```python
from build123d import *

# Parameters (mm, degrees)
F0_R     = 3
F1_DEPTH = 2
F2_DEPTH = 4
F4_DEPTH = 2
F5_DEPTH = 3


with BuildPart() as f1:
    # F0 (on Top) → F1 (new body)
    with BuildSketch(Plane.XY):
        with Locations((-50.25617, 22.832299)):
            Circle(F0_R)
        with BuildLine():
            Line((-57, -28.5), (43, -28.5))
            ThreePointArc((43, -28.5), (44.414214, -27.914214), (45, -26.5))
            Line((45, -26.5), (45, 26.5))
            ThreePointArc((45, 26.5), (44.414214, 27.914214), (43, 28.5))
            Line((43, 28.5), (-57, 28.5))
            Line((-57, 28.5), (-57, -28.5))
        make_face()
        with Locations((-50.25617, 22.832299)):
            Circle(F0_R, mode=Mode.SUBTRACT)
        with BuildLine():
            ThreePointArc((44, -26.5), (43.707107, -27.207107), (43, -27.5))
            Line((43, -27.5), (-43, -27.5))
            ThreePointArc((-43, -27.5), (-43.707107, -27.207107), (-44, -26.5))
            Line((-44, -26.5), (-44, 26.5))
            ThreePointArc((-44, 26.5), (-43.707107, 27.207107), (-43, 27.5))
            Line((-43, 27.5), (43, 27.5))
            ThreePointArc((43, 27.5), (43.707107, 27.207107), (44, 26.5))
            Line((44, 26.5), (44, -26.5))
        make_face(mode=Mode.SUBTRACT)
        with BuildLine():
            Line((-43, -27.5), (43, -27.5))
            ThreePointArc((43, -27.5), (43.707107, -27.207107), (44, -26.5))
            Line((44, -26.5), (44, 26.5))
            ThreePointArc((44, 26.5), (43.707107, 27.207107), (43, 27.5))
            Line((43, 27.5), (-43, 27.5))
            ThreePointArc((-43, 27.5), (-43.707107, 27.207107), (-44, 26.5))
            Line((-44, 26.5), (-44, -26.5))
            ThreePointArc((-44, -26.5), (-43.707107, -27.207107), (-43, -27.5))
        make_face()
    extrude(amount=F1_DEPTH)

    # F0 (on Top) → F2 (join)
    with BuildSketch(Plane.XY):
        with BuildLine():
            ThreePointArc((45, -26.5), (44.414214, -27.914214), (43, -28.5))
            Line((43, -28.5), (-57, -28.5))
            Line((-57, -28.5), (-57, -31.5))
            Line((-57, -31.5), (43, -31.5))
            ThreePointArc((43, -31.5), (46.535534, -30.035534), (48, -26.5))
            Line((48, -26.5), (48, 26.5))
            ThreePointArc((48, 26.5), (46.535534, 30.035534), (43, 31.5))
            Line((43, 31.5), (-57, 31.5))
            Line((-57, 31.5), (-57, 28.5))
            Line((-57, 28.5), (43, 28.5))
            ThreePointArc((43, 28.5), (44.414214, 27.914214), (45, 26.5))
            Line((45, 26.5), (45, -26.5))
        make_face()
    extrude(amount=F2_DEPTH)

    # F3 (on face) → F4 (cut)
    with BuildSketch(Plane.XY.offset(4)):
        Polygon((45, 3), (45, 0), (45, -3), (48, -3), (48, 0), (48, 3), align=None)
    extrude(amount=-F4_DEPTH, mode=Mode.SUBTRACT)

    # F0 (on Top) → F5 (cut)
    with BuildSketch(Plane.XY):
        with Locations((-50.25617, 22.832299)):
            Circle(F0_R)
    extrude(amount=F5_DEPTH, mode=Mode.SUBTRACT)


solid = f1.part
```
Input: part model. Units: mm. Frame: model coordinates. A direction names the side the tool comes from. Coordinates: 2 decimals unless noted, no trailing zeros. Loops run counter-clockwise (first coordinate to the right, second up) from the corner with the lowest first, then second, coordinate; pieces in that order, holes last. Notation, with made-up numbers: (65, 57.25) -> (115, 57.25) arc R10 cw to (115, 73.25) -> close; hole circle Ø1 at (54.25, -18). An arc over 180 degrees is marked (long way). Use a Markdown table: item, result.
1) Cut plane B-B (x = -46). Return the cut outline in (y, z), then the cut area to 3 significant figures.
Results found:
| item | result |
|---|---|
| outline | (-31.5, 0) -> (31.5, 0) -> (31.5, 4) -> (28.5, 4) -> (28.5, 2) -> (-28.5, 2) -> (-28.5, 4) -> (-31.5, 4) -> close |
| area | 138 mm2 |
2) Material intervals for line 1 along Y through (x, z) = (41.5, 2.15); line 2 along Z through (x, y) = (-11, 22); line 3 along X through (y, z) = (10, 2.25), sorted ascending. Write a range as from..to.
Results found:
| item | result |
|---|---|
| line 1 | y = -31.5..-28.5, 28.5..31.5 |
| line 2 | z = 0..2 |
| line 3 | x = 45..48 |
3) Cut plane A-A (z = 3.35). Return the cut outline in (x, y), then the cut area to 3 significant figures.
Results found:
| item | result |
|---|---|
| outline | (-57, -31.5) -> (43, -31.5) arc R5 ccw to (48, -26.5) -> (48, -3) -> (45, -3) -> (45, -26.5) arc R2 cw to (43, -28.5) -> (-57, -28.5) -> close; (-57, 28.5) -> (43, 28.5) arc R2 cw to (45, 26.5) -> (45, 3) -> (48, 3) -> (48, 26.5) arc R5 ccw to (43, 31.5) -> (-57, 31.5) -> close |
| area | 774 mm2 |
4) Cut plane C-C (y = 21). Return the cut outline in (x, z).
Results found:
| item | result |
|---|---|
| outline | (-57, 0) -> (-52.63, 0) -> (-52.63, 2) -> (-57, 2) -> close; (-47.88, 0) -> (48, 0) -> (48, 4) -> (45, 4) -> (45, 2) -> (-47.88, 2) -> close |
5) Access query for faces 5 (the flat face through (-6, 31.5, 2)), 6 (the flat face through (47, 3, 3)), 7 (the flat face through (-6, -28.5, 3)). Directions: +Z, -Z, +X, -X, +Y, -Y. A direction counts if a zero-diameter tool reaches every point of the face in a straight line with its end or side. Return the directions, or none.
Results found:
| item | result |
|---|---|
| face 5 | +Z, -Z, +X, -X, +Y |
| face 6 | +Z, +X, -X |
| face 7 | +Z, -X |
6) Contact query for flat-ended pins moving along their axis: pin 1 (1.6 mm diameter, centred on x = 46, z = 2.5, fed in from +Y); pin 2 (1.5 mm diameter, centred on x = -2, y = -15, fed in from +Z); pin 3 (5 mm diameter, centred on x = -50.26, y = 22.83, fed in from -Z); pin 4 (2 mm diameter, centred on x = 46.5, z = 3, fed in from -Y). Output: stop coordinate, or through.
Results found:
| item | result |
|---|---|
| pin 1 | stops at y = 30.99 |
| pin 2 | stops at z = 2 |
| pin 3 | passes through |
| pin 4 | stops at y = -30.83 |
7) Cut plane D-D (y = -8). Return the cut outline in (x, z), then the cut area to 3 significant figures.
Results found:
| item | result |
|---|---|
| outline | (-57, 0) -> (48, 0) -> (48, 4) -> (45, 4) -> (45, 2) -> (-57, 2) -> close |
| area | 216 mm2 |
8) Pull-direction query (Y, two-part tool) for faces 1 (the cylindrical face through (46.57, 30, 1.97)), 2 (the cylindrical face through (46.5, -30.07, 1.97)), 3 (the cylindrical face through (44.43, -27.9, 2.99)), 4 (the flat face through (45, 15, 3)); classes: released by +Y, released by -Y, zero draft, split by the parting line, or undercut.
Results found:
| item | result |
|---|---|
| face 1 | released by +Y |
| face 2 | released by -Y |
| face 3 | undercut |
| face 4 | undercut |
